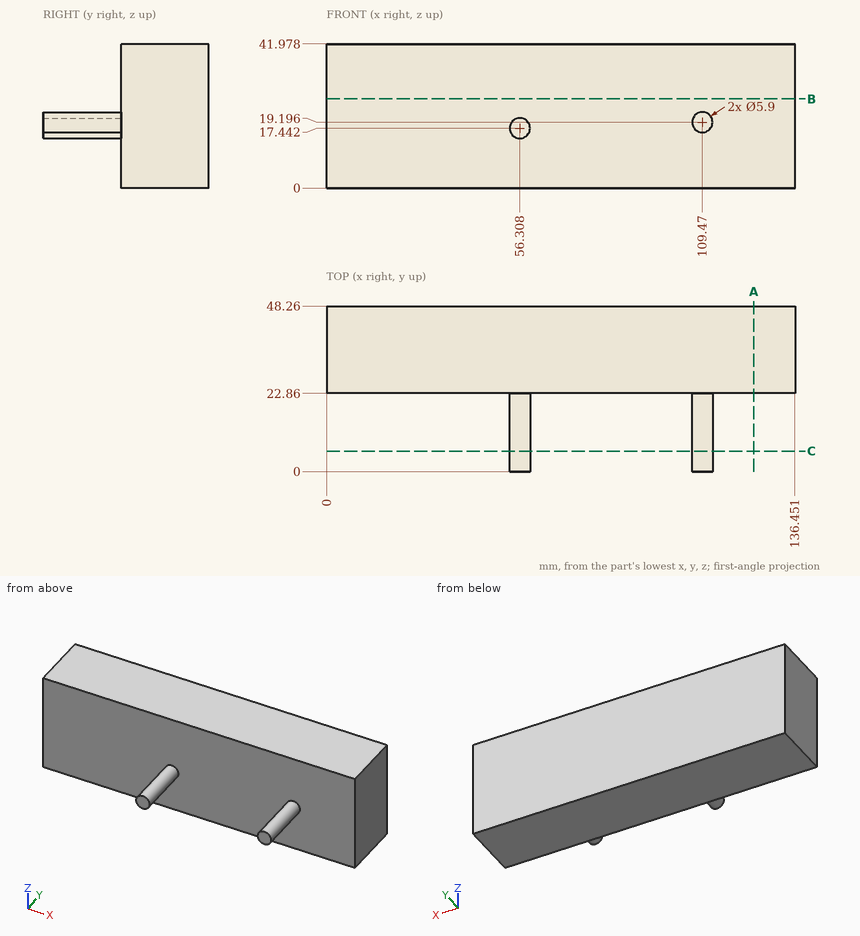
Input: dimensioned drawing with shaded views. Units: mm. Origin: part minimum x, y, z. Round coordinates to 2 decimals unless told otherwise and drop trailing zeros. Loops run counter-clockwise (first coordinate to the right, second up) from the corner with the lowest first, then second, coordinate; pieces in that order, holes last. Notation, with made-up numbers: M 24,41 L 41,41 A11 cw 41,62 Z; hole C 68,54.25 d11. An arc over 180 degrees is marked long. Answer in a Markdown table with one row per item. Add a question column.
1. Section B-B (z = 26). Output: boundary loops of the cut face in (x, y).
2. Section A-A (x = 124.5). Output: boundary loops of the cut face in (y, z).
3. Ray query, probe 1 along Y at (x, z) = (18, 23.5); probe 2 along X at (y, z) = (7, 20) (1 decimal); probe 3 along X at (y, z) = (17, 16.5) (1 decimal). Return the intervals inside material, ascending.
4. Section C-C (y = 6). Output: boundary loops of the cut face in (x, z), and give its area (3 significant figures).
5. Contact query for a flat-ended pin moving along its axis: pin 1 (4 mm diameter, centred on y = 20.5, z = 34, fed in from -X). Output: stop coordinate, or through.
Values follow:
| question | item | result |
|---|---|---|
| 1 | outline | M 0,22.86 L 136.45,22.86 L 136.45,48.26 L 0,48.26 Z |
| 2 | outline | M 22.86,0 L 48.26,0 L 48.26,41.98 L 22.86,41.98 Z |
| 3 | probe 1 | 22.86 to 48.26 |
| 3 | probe 2 | 54.8 to 57.8, 106.6 to 112.3 |
| 3 | probe 3 | 53.5 to 59.1, 108.3 to 110.7 |
| 4 | outline | C 56.31,17.44 d5.9; C 109.47,19.2 d5.9 |
| 4 | area | 54.7 mm^2 |
| 5 | pin 1 | through |
